from build123d import *

# Parameters (mm, degrees)
F2_SIZE = 30
F5_R    = 5


with BuildPart() as f1:
    # F0 (on Front) → F1 (revolve)
    with BuildSketch(Plane.XZ):
        Polygon((0, 0), (0, -101.104952), (200.569421, -100.49326), (200.569421, 20.011885), (165.090755, 20.011885), (160.197139, 0), align=None)
    revolve(axis=Axis((0, 0, -50.552476), (0, 0, 1)))

    # F2
    f2_edges = [f1.edges().sort_by_distance(p)[0] for p in [
        (-200.569421, 0, -100.49326),
    ]]
    chamfer(f2_edges, length=F2_SIZE)

    # F3 (on Front) → F4 (revolve)
    with BuildSketch(Plane.XZ):
        with BuildLine():
            Line((0, 0), (59.528868, 0))
            ThreePointArc((59.528868, 0), (0, 59.528868), (-59.528868, 0))
            Line((-59.528868, 0), (0, 0))
        make_face()
    revolve(axis=Axis((-29.764434, 0, 0), (-1, 0, 0)))

    # F5
    f5_edges = [f1.edges().sort_by_distance(p)[0] for p in [
        (-165.090755, 0, 20.011885),
        (-160.197139, 0, 0),
    ]]
    fillet(f5_edges, radius=F5_R)


solid = f1.part
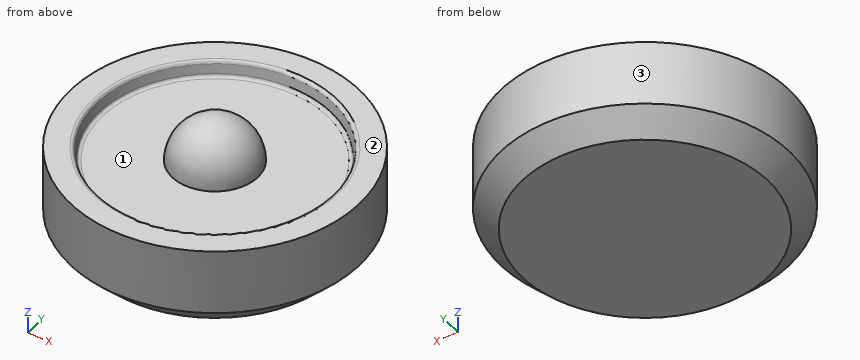
Here's how the part is built. I have some questions about the finished solid (model axes, mm). Face numbers are marked on the shaded views. Coordinates: 2 decimals unless noted, no trailing zeros. Write each loop counter-clockwise with the first axis right and the second up, starting at its lowest first coordinate (ties: lowest second). Pieces come first, ordered by that corner, then holes.
Item 1: If we mould it in two halves opening along Y, with no side actions, what happens to the marked faces 1, 2 and 3? For each: +Y half, -Y half, draft (parallel to the pull), parting line (faces both ways), or undercut.
Item 2: I want a section at A-A on z = -49. Write out the boundary of the cut face in (x, y), and give its area (3 significant figures).
Item 3: Will these pins go through, and if not, where does the flat tip stop? pin 1 (8 mm diameter, centred on y = -59, z = -54.5, fed in from -X); pin 2 (3 mm diameter, centred on y = -121.5, z = 3, fed in from -X); pin 3 (1.5 mm diameter, centred on x = 33.5, y = -49.5, fed in from -Z).
Item 4: If I drill on line 1 (Y direction, x = 1.5, z = -5); line 2 (Z direction, x = 134.5, y = 47); line 3 (Z direction, x = 20.5, y = 19), over which ranges is the centre line in solid material (lowest first)?
Findings below:
1. face 1: undercut
1. face 2: draft
1. face 3: parting line
2. outline: circle Ø401.14 at (0, 0)
2. area: 126,000 mm2
3. pin 1: stops at x = -192.88
3. pin 2: stops at x = -160.71
3. pin 3: stops at z = -100.92
4. line 1: y = -200.56 to 200.56
4. line 2: z = -100.67 to 0
4. line 3: z = -101.02 to 52.56
